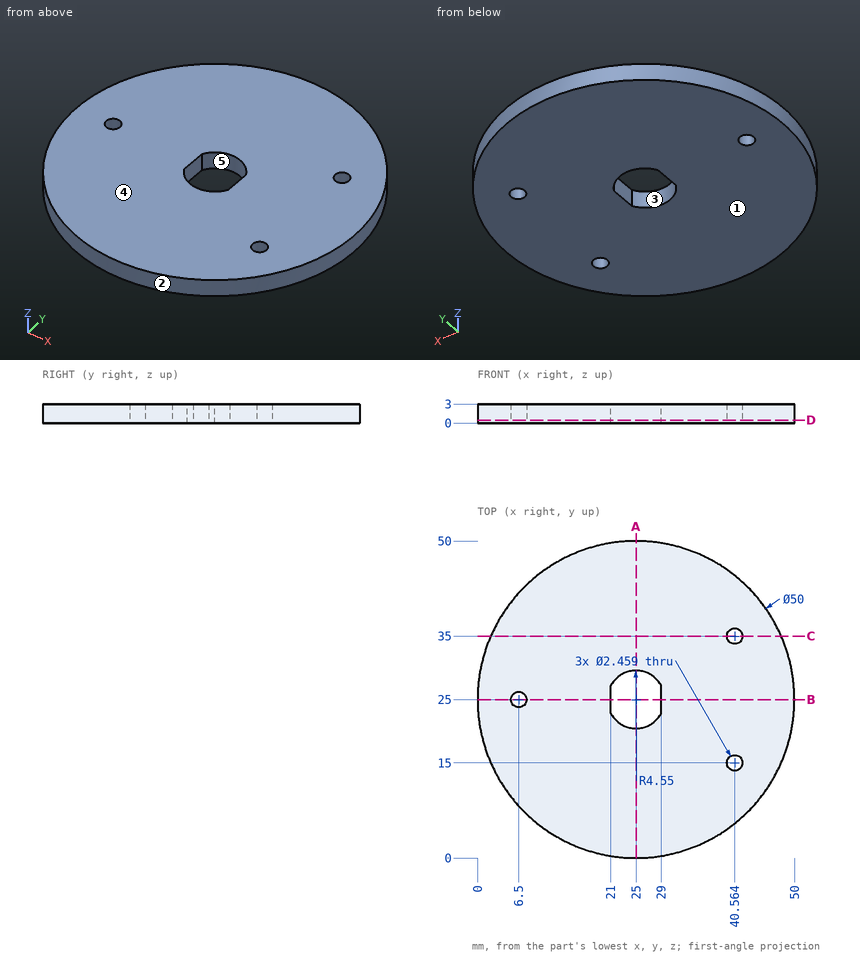
Check sheet for the drawn part. Datum: minimum x, y, z corner. Units: mm. A direction names the side the tool comes from. Round coordinates to 2 decimals unless told otherwise and drop trailing zeros. Order: outer loops, then holes, each group sorted by start corner. A loop starts at its lowest first (then second) coordinate and runs counter-clockwise, first axis right, second up.
(1) Scan lines: probe 1 along Y at (x, z) = (41, 0.5); probe 2 along X at (y, z) = (24.5, 1.3) (1 decimal); probe 3 along X at (y, z) = (27, 2.85). Record each from-to range of solid material in increasing order.
(2) Cross-section at B-B, the plane y = 25. Enter the section's corners in (x, z), and give its area (3 significant figures).
(3) Cross-section at A-A, the plane x = 25. Enter the section's corners in (y, z), and give its area (3 significant figures).
(4) Cross-section at C-C, the plane y = 35. Enter the section's corners in (x, z) (1 decimal), and give its area (3 significant figures).
(5) Cross-section at D-D, the plane z = 0.45. State how many separate pieces and enclosed holes the cut face has, and give its area (3 significant figures).
(6) Draft check along Y on the marked faces 1, 2 and 3. Enter one of: pulls with the +Y half, pulls with the -Y half, needs draft (parallel to the pull), parting line crosses it, or undercut.
(7) Access from +Z, -Z, +X, -X, +Y, -Y to the whole of each face (thin tool, end or side, straight path). Record for the marked faces 4 and 5.
(8) Go/stop test with flat-tipped pins: P1, Ø1.5, axis at x = 30, z = 2.5, coming from the +Y side; P2, Ø1, axis at x = 36.5, z = 0.5, coming from the +Y side. Record where each tip stops, or that it passes through.
Check sheet entries:
1. probe 1: y = 5.79 to 13.85, 16.15 to 33.85, 36.15 to 44.21
1. probe 2: x = 0 to 5.4, 7.6 to 21, 29 to 50
1. probe 3: x = 0.08 to 21, 29 to 49.92
2. outline: (0, 0) - (5.27, 0) - (5.27, 3) - (0, 3) - close; (7.73, 0) - (21, 0) - (21, 3) - (7.73, 3) - close; (29, 0) - (50, 0) - (50, 3) - (29, 3) - close
2. area: 119 mm2
3. outline: (0, 0) - (20.45, 0) - (20.45, 3) - (0, 3) - close; (29.55, 0) - (50, 0) - (50, 3) - (29.55, 3) - close
3. area: 123 mm2
4. outline: (2.1, 0) - (39.3, 0) - (39.3, 3) - (2.1, 3) - close; (41.8, 0) - (47.9, 0) - (47.9, 3) - (41.8, 3) - close
4. area: 130 mm2
5. separate pieces: 1
5. enclosed holes: 4
5. area: 1,890 mm2
6. face 1: needs draft
6. face 2: parting line crosses it
6. face 3: undercut
7. face 4: +Z, +X, -X, +Y, -Y
7. face 5: +Z, -Z
8. P1: stops at y = 49.64
8. P2: stops at y = 47.45
